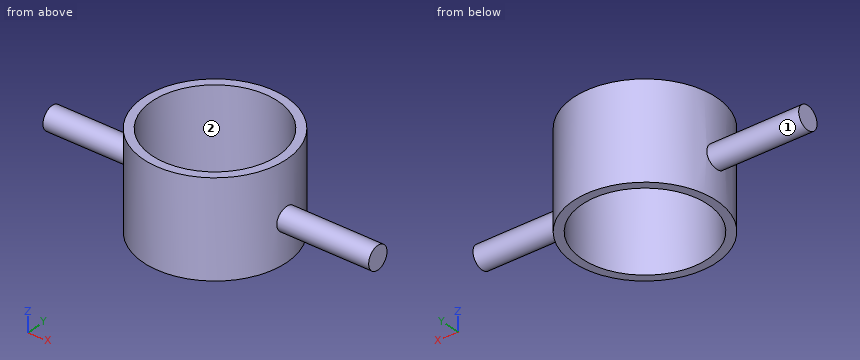
from build123d import *

# Parameters (mm, degrees)
F0_R     = 9.525
F1_DEPTH = 12.7
F2_R     = 8.382
F3_DEPTH = 25.4
F5_R     = 1.524
F6_DEPTH = 12.7


with BuildPart() as f1:
    # F0 (on Top) → F1 (new body)
    with BuildSketch(Plane.XY):
        Circle(F0_R)
    extrude(amount=F1_DEPTH)

    # F2 (on face) → F3 (cut)
    with BuildSketch(Plane.XY.offset(12.7)):
        Circle(F2_R)
    extrude(amount=-F3_DEPTH, mode=Mode.SUBTRACT)

    # F5 (on offset) → F6 (join)
    with BuildSketch(Plane.YZ.offset(8.89)):
        with Locations((0, 5.393751)):
            Circle(F5_R)
    extrude(amount=F6_DEPTH)

    # F7: F1 across plane


with BuildPart() as f1_1:
    add(f1.part)
    add(f1.part.mirror(Plane.YZ))


solid = f1_1.part
Here's how the part is built. I have some questions about the finished solid (model axes, mm). Face numbers are marked on the shaded views. Round coordinates to 2 decimals unless told otherwise and drop trailing zeros. Write each loop counter-clockwise with the first axis right and the second up, starting at its lowest first coordinate (ties: lowest second). Pieces come first, ordered by that corner, then holes.
1. If we mould it in two halves opening along Y, with no side actions, what happens to the marked faces 1 and 2? For each: released by +Y, released by -Y, zero draft, split by the parting line, or undercut.
2. Will these pins go through, and if not, where does the flat tip stop? pin 1 Ø2 at (y, z) = (2, 10.5) entering from -X; pin 2 Ø4 at (y, z) = (-6, 3) entering from -X; pin 3 Ø1 at (y, z) = (2, 4.5) entering from +X.
3. Suppose I cut it at D-D (x = -7). List the corners of the cut face in (y, z) for me.
4. Suppose I cut it at C-C (z = 2.5). List the corners of the cut face in (x, y) for me (3 decimals), and give its area (3 significant figures).
5. Suppose I cut it at B-B (y = 0). List the corners of the cut face in (x, z) for me (3 decimals).
6. Suppose I cut it at A-A (x = 0). List the corners of the cut face in (y, z) for me (3 decimals), and give its area (3 significant figures).
7. I need wall thicknesses on L1, parallel to Y at x = 0, z = 5.25 (3 decimals); L2, parallel to X at y = -0.25, z = 7.5; L3, parallel to X at y = -2, z = 10.5. Which ranges of each line are inside material? Lowest first, please.
Answer sheet:
1. face 1: split by the parting line
1. face 2: undercut
2. pin 1: stops at x = -9.47
2. pin 2: stops at x = -8.64
2. pin 3: stops at x = 9.41
3. outline: (-6.46, 0) - (-4.61, 0) - (-4.61, 12.7) - (-6.46, 12.7) - close; (4.61, 0) - (6.46, 0) - (6.46, 12.7) - (4.61, 12.7) - close
4. outline: circle Ø19.05 at (0, 0); hole circle Ø16.764 at (0, 0)
4. area: 64.3 mm2
5. outline: (-21.59, 3.87) - (-9.525, 3.87) - (-9.525, 0) - (-8.382, 0) - (-8.382, 12.7) - (-9.525, 12.7) - (-9.525, 6.918) - (-21.59, 6.918) - close; (8.382, 0) - (9.525, 0) - (9.525, 3.87) - (21.59, 3.87) - (21.59, 6.918) - (9.525, 6.918) - (9.525, 12.7) - (8.382, 12.7) - close
6. outline: (-9.525, 0) - (-8.382, 0) - (-8.382, 12.7) - (-9.525, 12.7) - close; (8.382, 0) - (9.525, 0) - (9.525, 12.7) - (8.382, 12.7) - close
6. area: 29.0 mm2
7. L1: y = -9.525 to -8.382, 8.382 to 9.525
7. L2: x = -9.52 to -8.38, 8.38 to 9.52
7. L3: x = -9.31 to -8.14, 8.14 to 9.31
